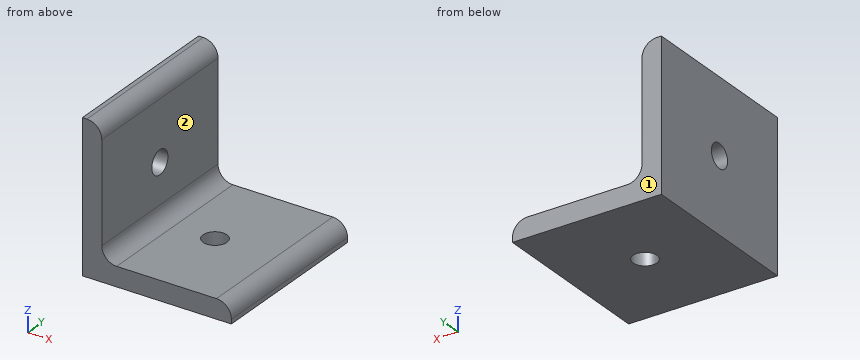
```python
from build123d import *

# Parameters (mm, degrees)
BOSS_EXTRUDE1_DEPTH = 29.21
FILLET1_R           = 2.54
SKETCH2_R           = 2.032
CUT_EXTRUDE1_DEPTH  = 26.4
SKETCH3_R           = 2.032
CUT_EXTRUDE2_DEPTH  = 26.4


with BuildPart() as part:
    # Sketch1 → Boss-Extrude1 (new body)
    with BuildSketch(Plane(origin=(0, 0, 0), x_dir=(1, 0, 0), z_dir=(0, 1, 0))):
        Polygon((0, 0), (0, -25.4), (3.302, -25.4), (3.302, -3.302), (25.4, -3.302), (25.4, 0), align=None)
    extrude(amount=BOSS_EXTRUDE1_DEPTH)

    # Fillet1
    fillet1_edges = [part.edges().sort_by_distance(p)[0] for p in [
        (25.4, 14.605, 3.302),
        (3.302, 14.605, 3.302),
        (3.302, 14.605, 25.4),
    ]]
    fillet(fillet1_edges, radius=FILLET1_R)

    # Sketch2 → Cut-Extrude1 (cut, through all)
    with BuildSketch(Plane.ZY):
        with Locations((12.7, 14.605)):
            Circle(SKETCH2_R)
    extrude(amount=-CUT_EXTRUDE1_DEPTH, mode=Mode.SUBTRACT)

    # Sketch3 → Cut-Extrude2 (cut, through all)
    with BuildSketch(Plane(origin=(0, 0, 0), x_dir=(-1, 0, 0), z_dir=(0, 0, -1))):
        with Locations((-12.7, 14.605)):
            Circle(SKETCH3_R)
    extrude(amount=-CUT_EXTRUDE2_DEPTH, mode=Mode.SUBTRACT)


solid = part.part
```
Input: part model. Units: mm. Frame: model coordinates. Face numbers are marked on the shaded views. A direction names the side the tool comes from. Coordinates: 2 decimals unless noted, no trailing zeros. Loops run counter-clockwise (first coordinate to the right, second up) from the corner with the lowest first, then second, coordinate; pieces in that order, holes last. Notation, with made-up numbers: M 75.25,36 L 106.25,36 A30 cw 106.25,68 Z; hole C 46,-33 d3. An arc over 180 degrees is marked long. One line per item, written item: value.
(1) Reachability of the marked faces 1 and 2 from +Z, -Z, +X, -X, +Y, -Y: full face, straight path, thin tool, end or side. Return the list, or none.
Filled in:
face 1: +Z, -Z, +X, -X, +Y
face 2: +Z, +X, +Y, -Y
(2) Section C-C (y = 6.5). Output: boundary loops of the cut face in (x, z), and give its area (3 significant figures).
Filled in:
outline: M 0,0 L 25.4,0 L 25.4,0.76 A2.54 ccw 22.86,3.3 L 5.84,3.3 A2.54 cw 3.3,5.84 L 3.3,22.86 A2.54 ccw 0.76,25.4 L 0,25.4 Z
area: 155 mm^2
(3) Line query: line 1 along Y through (x, z) = (2.05, 12.7); line 2 along X through (y, z) = (26.25, 7.75). Output: solid intervals per line, ascending. Write a range as from..to.
Filled in:
line 1: 0..12.57, 16.64..29.21
line 2: 0..3.3
(4) Pin query (flat end, axial travel): pin 1 (5 mm diameter, centred on x = 12.5, y = 19.5, fed in from +Z); pin 2 (12 mm diameter, centred on y = 17, z = 11, fed in from +X); pin 3 (3.5 mm diameter, centred on y = 14.605, z = 12.7, fed in from +X); pin 4 (13.5 mm diameter, centred on y = 10, z = 13.5, fed in from +X). Return the tip coordinate at first contact, or that it passes through.
Filled in:
pin 1: z = 3.3
pin 2: x = 3.45
pin 3: through
pin 4: x = 3.3
(5) Section B-B (x = 12.7). Output: boundary loops of the cut face in (y, z), and give its area (3 significant figures).
Filled in:
outline: M 0,0 L 12.57,0 L 12.57,3.3 L 0,3.3 Z; M 16.64,0 L 29.21,0 L 29.21,3.3 L 16.64,3.3 Z
area: 83.0 mm^2
(6) Section D-D (z = 2.75). Output: boundary loops of the cut face in (x, y) (3 decimals), and give its area (3 significant figures).
Filled in:
outline: M 0,0 L 24.441,0 L 24.441,29.21 L 0,29.21 Z; hole C 12.7,14.605 d4.064
area: 701 mm^2
(7) Section A-A (z = 12.7). Output: boundary loops of the cut face in (x, y), and give its area (3 significant figures).
Filled in:
outline: M 0,0 L 3.3,0 L 3.3,12.57 L 0,12.57 Z; M 0,16.64 L 3.3,16.64 L 3.3,29.21 L 0,29.21 Z
area: 83.0 mm^2
